```python
from build123d import *

# Parameters (mm, degrees)
SKETCH_W               = 280
SKETCH_H               = 8
PAD_DEPTH              = 1.65
SKETCH001_W            = 2
SKETCH001_H            = 5
POCKET_DEPTH           = 5
LINEARPATTERN_COUNT    = 15
LINEARPATTERN_PITCH    = 17
SKETCH002_W            = 5
SKETCH002_H            = 4
POCKET001_DEPTH        = 5
LINEARPATTERN001_COUNT = 2
LINEARPATTERN001_PITCH = 275
SKETCH003_W            = 8
SKETCH003_H            = 1.65
SKETCH003_W_2          = 18
PAD001_DEPTH           = 5


with BuildPart() as part:
    # Sketch → Pad (new body)
    with BuildSketch(Plane.XY):
        Rectangle(SKETCH_W, SKETCH_H)
    extrude(amount=PAD_DEPTH)

    # Sketch001 (on Face6 of Pad) → Pocket (cut)
    with BuildSketch(Plane.XY.offset(1.65)):
        with Locations((-119, 1.5)):
            Rectangle(SKETCH001_W, SKETCH001_H)
    pocket = extrude(amount=-POCKET_DEPTH, mode=Mode.SUBTRACT)

    # LinearPattern: Pocket ×15
    with Locations(*[(i * LINEARPATTERN_PITCH, 0, 0) for i in range(1, LINEARPATTERN_COUNT)]):
        add(pocket, mode=Mode.SUBTRACT)

    # Sketch002 (on Face4 of LinearPattern) → Pocket001 (cut)
    with BuildSketch(Plane.XY.offset(1.65)):
        with Locations((-137.5, -2)):
            Rectangle(SKETCH002_W, SKETCH002_H)
    pocket001 = extrude(amount=-POCKET001_DEPTH, mode=Mode.SUBTRACT)

    # LinearPattern001: Pocket001 ×2
    with Locations(*[(i * LINEARPATTERN001_PITCH, 0, 0) for i in range(1, LINEARPATTERN001_COUNT)]):
        add(pocket001, mode=Mode.SUBTRACT)

    # Sketch003 (on Face68 of LinearPattern001) → Pad001 (join)
    with BuildSketch(Plane.XZ.offset(4)):
        with Locations((-81, 0.825)):
            Rectangle(SKETCH003_W, SKETCH003_H)
        with Locations((0, 0.825)):
            Rectangle(SKETCH003_W_2, SKETCH003_H)
        with Locations((81, 0.825)):
            Rectangle(SKETCH003_W, SKETCH003_H)
    extrude(amount=PAD001_DEPTH)


solid = part.part
```
Can you work these out from the model? Positions are in its coordinate system, mm. Coordinates: 2 decimals unless noted, no trailing zeros. Loops run counter-clockwise (first coordinate to the right, second up) from the corner with the lowest first, then second, coordinate; pieces in that order, holes last. Notation, with made-up numbers: (-2.5, 6.25) - (21.5, 6.25) arc R13 ccw to (21.5, 18.25) - close; hole circle Ø5 at (86, 43). An arc over 180 degrees is marked (long way). Answer as CSV lines item,"result". Start each with the question number.
1) For pin 1 (0.5 mm diameter, centred on x = -30, z = 1, fed in from -Y); pin 2 (0.8 mm diameter, centred on x = -85, z = 0.5, fed in from +Y), each with a flat end and sliding along its axis, tell me the tip position at first contact or that it passes through.
2) I need wall thicknesses on line 1 (X direction, y = -5, z = 0.9); line 2 (Y direction, x = 128, z = 1.5); line 3 (Y direction, x = 0.5, z = 1.15). Which ranges of each line are inside material? Lowest first, please. Write a range as from..to.
3) Suppose I cut it at A-A (x = -47.5). Please give me the cut outline in (y, z).
Check result:
1,pin 1,"stops at y = -4"
1,pin 2,"stops at y = -1"
2,line 1,"x = -85..-77, -9..9, 77..85"
2,line 2,"y = -4..4"
2,line 3,"y = -9..-1"
3,outline,"(-4, 0) - (4, 0) - (4, 1.65) - (-4, 1.65) - close"
